Input: dimensioned drawing with shaded views. Units: mm. Origin: part minimum x, y, z. A direction names the side the tool comes from. Give positions to 0.01 mm unless a question says otherwise; leave off trailing zeros. Order: outer loops, then holes, each group sorted by start corner. A loop starts at its lowest first (then second) coordinate and runs counter-clockwise, first axis right, second up. Notation, with made-up numbers: (-11.5, -21.75) -> (25.5, -21.75) arc R20 cw to (25.5, -12.75) -> close; hole circle Ø7 at (50.25, -8.75). An arc over 180 degrees is marked (long way). Use CSV: the item, a comma, the result in double quotes.
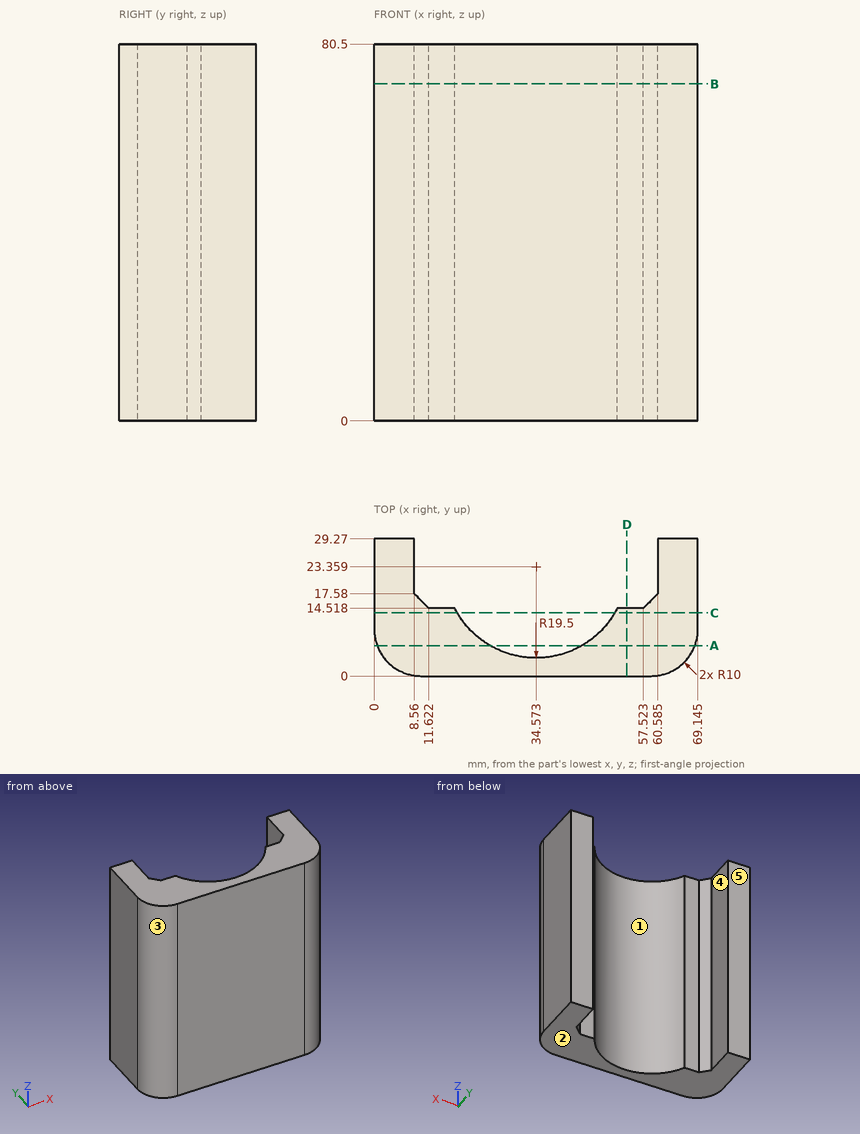
1. Section query B-B on z = 72. Return loops of the section in (x, y) (1 decimal).
Answer below:
outline,"(0, 10) arc R10 ccw to (10, 0) -> (59.1, 0) arc R10 ccw to (69.1, 10) -> (69.1, 29.3) -> (60.6, 29.3) -> (60.6, 17.6) -> (57.5, 14.5) -> (52, 14.5) arc R19.5 cw to (17.2, 14.5) -> (11.6, 14.5) -> (8.6, 17.6) -> (8.6, 29.3) -> (0, 29.3) -> close"
2. Ray query, line 1 along X through (y, z) = (24, 26.5) (1 decimal); line 2 along X through (y, z) = (12, 53) (1 decimal); line 3 along X through (y, z) = (2, 9) (1 decimal). Return the intervals inside material, ascending.
Answer below:
line 1,"x = 0 to 8.6, 60.6 to 69.1"
line 2,"x = 0 to 18.7, 50.4 to 69.1"
line 3,"x = 4 to 65.1"
3. Mould query, pull axis X, two halves, no side actions, for the marked faces 1, 2 and 3. Classes: released by +X, released by -X, zero draft, split by the parting line, or undercut.
Answer below:
face 1,"undercut"
face 2,"zero draft"
face 3,"released by -X"
4. Pin query (flat end, axial travel): P1, Ø4.5, axis at x = 54, z = 48, coming from the +Y side. Return the tip coordinate at first contact, or that it passes through.
Answer below:
P1,"stops at y = 14.52"
5. Section query D-D on x = 54. Return loops of the section in (y, z).
Answer below:
outline,"(0, 0) -> (14.52, 0) -> (14.52, 80.5) -> (0, 80.5) -> close"
6. Section query C-C on y = 13.5. Return loops of the section in (x, z) (1 decimal), plus the area to 3 significant figures.
Answer below:
outline,"(0, 0) -> (17.7, 0) -> (17.7, 80.5) -> (0, 80.5) -> close; (51.4, 0) -> (69.1, 0) -> (69.1, 80.5) -> (51.4, 80.5) -> close"
area,"2,860 mm²"
7. Access query for the marked faces 4 and 5. Directions: +Z, -Z, +X, -X, +Y, -Y. A direction counts if a zero-diameter tool reaches every point of the face in a straight line with its end or side. Return the directions, or none.
Answer below:
face 4,"+Z, -Z, +Y"
face 5,"+Z, -Z, +X, -X, +Y"
8. Section query A-A on y = 6.5. Return loops of the section in (x, z), plus the area to 3 significant figures.
Answer below:
outline,"(0.63, 0) -> (24.77, 0) -> (24.77, 80.5) -> (0.63, 80.5) -> close; (44.37, 0) -> (68.51, 0) -> (68.51, 80.5) -> (44.37, 80.5) -> close"
area,"3,890 mm²"
